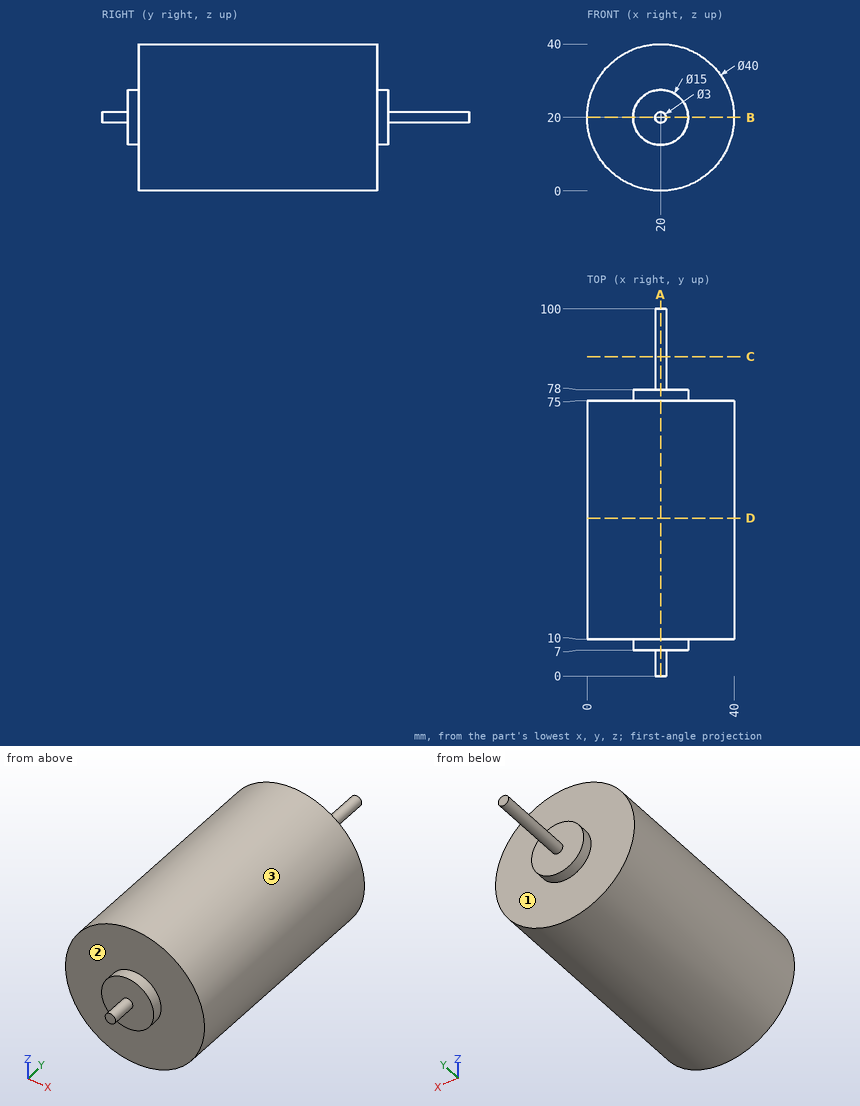
For this review, use the dimensioned drawing (mm, ordinates from the lowest corner) and the shaded views. A direction names the side the tool comes from. Round coordinates to 2 decimals unless told otherwise and drop trailing zeros. Write each loop counter-clockwise with the first axis right and the second up, starting at its lowest first coordinate (ties: lowest second). Pieces come first, ordered by that corner, then holes. Notation, with made-up numbers: (76.5, -31.5) -> (129.5, -31.5) arc R12 cw to (129.5, -11.5) -> close; hole circle Ø1 at (-20, 9.5). An arc over 180 degrees is marked (long way). Use one line per item in the form item = value.
Q1. To check wall thickness, follow probe 1 along Y at (x, z) = (29, 24); probe 2 along X at (y, z) = (43, 20); probe 3 along X at (y, z) = (29, 22). State the ranges of each line that lie inside material, in increasing order. Write a range as from..to.
Resolved:
probe_1 = 10..75
probe_2 = 0..40
probe_3 = 0.1..39.9
Q2. Consider section A-A (x = 20). State the section outline as (y, z) points.
Resolved:
outline = (0, 18.5) -> (7, 18.5) -> (7, 12.5) -> (10, 12.5) -> (10, 0) -> (75, 0) -> (75, 12.5) -> (78, 12.5) -> (78, 18.5) -> (100, 18.5) -> (100, 21.5) -> (78, 21.5) -> (78, 27.5) -> (75, 27.5) -> (75, 40) -> (10, 40) -> (10, 27.5) -> (7, 27.5) -> (7, 21.5) -> (0, 21.5) -> close
Q3. Machinability: for the marked faces 1, 2 and 3, which of the approach directions +Z, -Z, +X, -X, +Y, -Y give a long, thin tool a straight path to every point of the face, cutting with its end or side? Answer none if there is none.
Resolved:
face_1 = +Y
face_2 = -Y
face_3 = +Y, -Y
Q4. Consider section D-D (y = 43). State the section outline as (x, z) points, then the cut area to 3 significant figures.
Resolved:
outline = circle Ø40 at (20, 20)
area = 1,260 mm²
Q5. Clearance check with flat-ended pins moving along their axes: pin 1 Ø8 at (y, z) = (51.5, 19) entering from -X; pin 2 Ø3 at (x, z) = (17, 5.5) entering from +Y; pin 3 Ø4 at (x, z) = (25, 11) entering from -Y. State where each tip first meets the part, or that it passes through.
Resolved:
pin_1 = 0
pin_2 = 75
pin_3 = 10
Q6. Consider section C-C (y = 87). State the section outline as (x, z) points, then the cut area to 3 significant figures.
Resolved:
outline = circle Ø3 at (20, 20)
area = 7.07 mm²
Q7. Consider section B-B (z = 20). State the section outline as (x, y) points, then the cut area to 3 significant figures.
Resolved:
outline = (0, 10) -> (12.5, 10) -> (12.5, 7) -> (18.5, 7) -> (18.5, 0) -> (21.5, 0) -> (21.5, 7) -> (27.5, 7) -> (27.5, 10) -> (40, 10) -> (40, 75) -> (27.5, 75) -> (27.5, 78) -> (21.5, 78) -> (21.5, 100) -> (18.5, 100) -> (18.5, 78) -> (12.5, 78) -> (12.5, 75) -> (0, 75) -> close
area = 2,780 mm²
